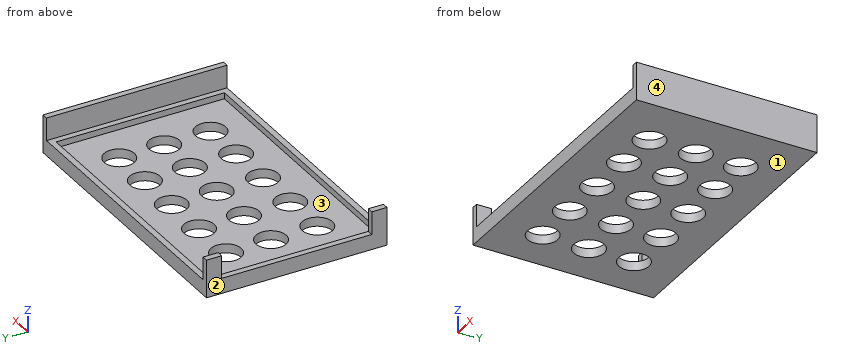
from build123d import *

# Parameters (mm, degrees)
F0_W      = 95.25
F0_H      = 60.325
F1_DEPTH  = 3.048
F2_W      = 2.032
F2_H      = 60.325
F3_DEPTH  = 9.652
F4_W      = 2.032
F4_H      = 5.08
F5_DEPTH  = 9.652
F6_W      = 2.032
F6_H      = 5.08
F7_DEPTH  = 9.652
F8_W      = 91.186
F8_H      = 2.027074
F8_H_2    = 2.032
F9_DEPTH  = 2.032
F10_W     = 2.032
F10_H     = 50.165
F11_DEPTH = 2.032
F12_W     = 2.032
F12_H     = 56.265926
F13_DEPTH = 2.032
F14_R     = 5.08
F15_DEPTH = 25.4


with BuildPart() as f1:
    # F0 (on Top) → F1 (new body)
    with BuildSketch(Plane.XY):
        with Locations((-6.869216, -18.085686)):
            Rectangle(F0_W, F0_H)
    extrude(amount=F1_DEPTH)

    # F2 (on face) → F3 (join)
    with BuildSketch(Plane.XY.offset(3.048)):
        with Locations((39.739784, -18.085686)):
            Rectangle(F2_W, F2_H)
    extrude(amount=F3_DEPTH)

    # F4 (on face) → F5 (join)
    with BuildSketch(Plane.XY.offset(3.048)):
        with Locations((-53.478216, -45.708186)):
            Rectangle(F4_W, F4_H)
    extrude(amount=F5_DEPTH)

    # F6 (on face) → F7 (join)
    with BuildSketch(Plane.XY.offset(3.048)):
        with Locations((-53.478216, 9.536814)):
            Rectangle(F6_W, F6_H)
    extrude(amount=F7_DEPTH)

    # F8 (on face) → F9 (join)
    with BuildSketch(Plane.XY.offset(3.048)):
        with Locations((-6.869216, 11.063277)):
            Rectangle(F8_W, F8_H)
        with Locations((-6.869216, -47.232186)):
            Rectangle(F8_W, F8_H_2)
    extrude(amount=F9_DEPTH)

    # F10 (on face) → F11 (join)
    with BuildSketch(Plane.XY.offset(3.048)):
        with Locations((-53.478216, -18.085686)):
            Rectangle(F10_W, F10_H)
    extrude(amount=F11_DEPTH)

    # F12 (on face) → F13 (join)
    with BuildSketch(Plane.XY.offset(3.048)):
        with Locations((37.707784, -18.083223)):
            Rectangle(F12_W, F12_H)
    extrude(amount=F13_DEPTH)

    # F14 (on face) → F15 (cut)
    with BuildSketch(Plane.XY.offset(3.048)):
        with Locations((-39.531879, -3.051191)):
            Circle(F14_R)
        with Locations((-23.761189, -3.051191)):
            Circle(F14_R)
        with Locations((-7.885216, -3.051191)):
            Circle(F14_R)
        with Locations((7.780211, -3.051191)):
            Circle(F14_R)
        with Locations((22.709807, -3.051191)):
            Circle(F14_R)
        with Locations((22.709807, -18.083223)):
            Circle(F14_R)
        with Locations((7.780211, -18.083223)):
            Circle(F14_R)
        with Locations((-7.885216, -18.083223)):
            Circle(F14_R)
        with Locations((-23.761189, -18.083223)):
            Circle(F14_R)
        with Locations((-39.531879, -18.083223)):
            Circle(F14_R)
        with Locations((-39.531879, -33.541203)):
            Circle(F14_R)
        with Locations((-23.761189, -33.541203)):
            Circle(F14_R)
        with Locations((-7.885216, -33.541203)):
            Circle(F14_R)
        with Locations((22.709807, -33.541203)):
            Circle(F14_R)
        with Locations((7.780211, -33.541203)):
            Circle(F14_R)
    extrude(amount=-F15_DEPTH, mode=Mode.SUBTRACT)


solid = f1.part
Check sheet for the modelled part. Datum: model origin and axes. Units: mm. Face numbers are marked on the shaded views. Round coordinates to 2 decimals unless told otherwise and drop trailing zeros. Loops run counter-clockwise (first coordinate to the right, second up) from the corner with the lowest first, then second, coordinate; pieces in that order, holes last.
1. Gauge pin test, flat ends, axial feed: pin 1 Ø4 at (y, z) = (-26, 9.5) entering from -X; pin 2 Ø11.5 at (x, y) = (-7.89, -3.05) entering from +Z; pin 3 Ø1 at (x, y) = (-53.5, -7.5) entering from +Z. Record the tip position at first contact, or that the pin passes through.
2. Scan lines: probe 1 along Y at (x, z) = (3.5, 1.75); probe 2 along X at (y, z) = (-36.5, 1.5); probe 3 along X at (y, z) = (-21.5, 4.5). Record each from-to range of solid material in increasing order.
3. Sectioned sample at D-D on y = -42. Record the boundary of the cut face in (x, z).
4. Sectioned sample at B-B on x = -46. Record the boundary of the cut face in (y, z).
5. Mould release check, pull along X, two halves, no side actions. Record for the marked faces 1, 2, 3 and 4: released by +X, released by -X, zero draft, split by the parting line, or undercut.
6. Sectioned sample at A-A on z = 10.75. Record the boundary of the cut face in (x, y).
7. Sectioned sample at C-C on x = -23. Record the boundary of the cut face in (y, z), and give its area (3 significant figures).
Recorded:
1. pin 1: stops at x = 38.72
1. pin 2: stops at z = 3.05
1. pin 3: stops at z = 5.08
2. probe 1: y = -48.25 to -36.28, -30.81 to -20.82, -15.35 to -5.79, -0.32 to 12.08
2. probe 2: x = -54.49 to -43.66, -35.4 to -27.89, -19.63 to -12.01, -3.76 to 3.65, 11.91 to 18.58, 26.84 to 40.76
2. probe 3: x = -54.49 to -52.46, 36.69 to 40.76
3. outline: (-54.49, 0) - (40.76, 0) - (40.76, 12.7) - (38.72, 12.7) - (38.72, 5.08) - (36.69, 5.08) - (36.69, 3.05) - (-52.46, 3.05) - (-52.46, 5.08) - (-54.49, 5.08) - close
4. outline: (-48.25, 0) - (12.08, 0) - (12.08, 5.08) - (10.05, 5.08) - (10.05, 3.05) - (-46.22, 3.05) - (-46.22, 5.08) - (-48.25, 5.08) - close
5. face 1: zero draft
5. face 2: released by -X
5. face 3: undercut
5. face 4: released by +X
6. outline: (-54.49, -48.25) - (-52.46, -48.25) - (-52.46, -43.17) - (-54.49, -43.17) - close; (-54.49, 7) - (-52.46, 7) - (-52.46, 12.08) - (-54.49, 12.08) - close; (38.72, -48.25) - (40.76, -48.25) - (40.76, 12.08) - (38.72, 12.08) - close
7. outline: (-48.25, 0) - (-38.56, 0) - (-38.56, 3.05) - (-46.22, 3.05) - (-46.22, 5.08) - (-48.25, 5.08) - close; (-28.52, 0) - (-23.11, 0) - (-23.11, 3.05) - (-28.52, 3.05) - close; (-13.06, 0) - (-8.07, 0) - (-8.07, 3.05) - (-13.06, 3.05) - close; (1.97, 0) - (12.08, 0) - (12.08, 5.08) - (10.05, 5.08) - (10.05, 3.05) - (1.97, 3.05) - close
7. area: 100 mm2
